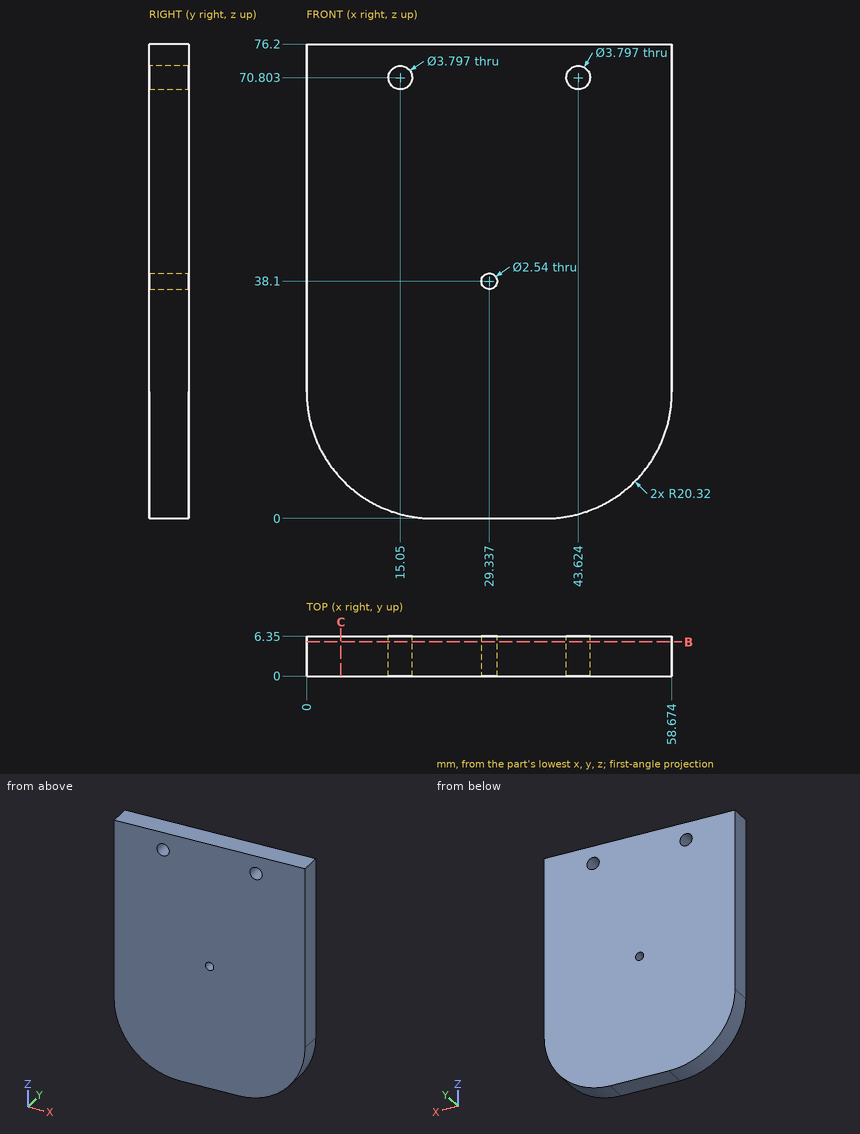
Geometry check sheet. Reference: drawing and pictorial views, mm from the part's lowest x, y, z. Round coordinates to 2 decimals unless told otherwise and drop trailing zeros. Write each loop counter-clockwise with the first axis right and the second up, starting at its lowest first coordinate (ties: lowest second). Pieces come first, ordered by that corner, then holes. Notation, with made-up numbers: (9, 50) -> (38, 50) arc R10 cw to (38, 65) -> close; hole circle Ø7 at (21.25, 84.5). An arc over 180 degrees is marked (long way). Put each result on its own line as item: value.
1) Cross-section at C-C, the plane x = 5.5. Enter the section's corners in (y, z).
Recorded:
outline: (0, 6.42) -> (6.35, 6.42) -> (6.35, 76.2) -> (0, 76.2) -> close
2) Cross-section at B-B, the plane y = 5.5. Give the number of separate pieces and of enclosed holes in the cut face, plus the area to 3 significant figures.
Recorded:
separate pieces: 1
enclosed holes: 3
area: 4,270 mm2
3) Thickness scan on probe 1 along X at (y, z) = (6, 71) (1 decimal); probe 2 along Z at (x, y) = (39, 0.5); probe 3 along Z at (x, y) = (12, 6). Record the ranges inside material, lowest first. Write a range as from..to.
Recorded:
probe 1: x = 0..13.2, 16.9..41.7, 45.5..58.7
probe 2: z = 0.01..76.2
probe 3: z = 1.78..76.2
